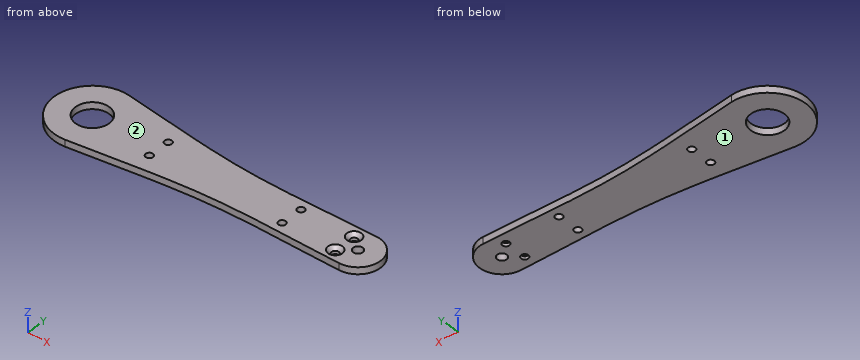
from build123d import *

# Parameters (mm, degrees)
SKETCH1_R           = 7.5
SKETCH1_R_2         = 2.125
SKETCH1_R_3         = 1.6
BOSS_EXTRUDE1_DEPTH = 3
SKETCH2_R           = 1.6
CUT_EXTRUDE1_DEPTH  = 79.91134278
CHAMFER1_SIZE       = 1.6


with BuildPart() as part:
    # Sketch1 → Boss-Extrude1 (new body)
    with BuildSketch(Plane.XY):
        with BuildLine():
            ThreePointArc((-57.956829007, 16.876772567), (-77, 0), (-57.956829007, -16.876772567))
            add(Edge.make_bspline(
                [(60, -10), (39.938279517, -10), (0.415985338, -7.693613776), (-38.598478023, -14.486949791), (-57.956829007, -16.876772567)],
                knots=[0, 0, 0, 0, 0.506913544, 1, 1, 1, 1], degree=3))
            ThreePointArc((60, -10), (70, 0), (60, 10))
            add(Edge.make_bspline(
                [(60, 10), (39.938279517, 10), (0.415985338, 7.693613776), (-38.598478023, 14.486949791), (-57.956829007, 16.876772567)],
                knots=[0, 0, 0, 0, 0.506913544, 1, 1, 1, 1], degree=3))
        make_face()
        with Locations((-60, 0)):
            Circle(SKETCH1_R, mode=Mode.SUBTRACT)
        with Locations(Location((60, 0, 0), (0, 0, 180))):
            Circle(SKETCH1_R_2, mode=Mode.SUBTRACT)
        with Locations((-30, 5)):
            Circle(SKETCH1_R_3, mode=Mode.SUBTRACT)
        with Locations((30, 5)):
            Circle(SKETCH1_R_3, mode=Mode.SUBTRACT)
        with Locations((30, -5)):
            Circle(SKETCH1_R_3, mode=Mode.SUBTRACT)
        with Locations((-30, -5)):
            Circle(SKETCH1_R_3, mode=Mode.SUBTRACT)
    extrude(amount=BOSS_EXTRUDE1_DEPTH)

    # Sketch2 → Cut-Extrude1 (cut, through all)
    with BuildSketch(Plane.XY.offset(3)):
        with Locations((54, 5)):
            Circle(SKETCH2_R)
        with Locations(Location((54, -5, 0), (0, 0, 180))):
            Circle(SKETCH2_R)
    extrude(amount=-CUT_EXTRUDE1_DEPTH, mode=Mode.SUBTRACT)

    # Chamfer1
    chamfer1_edges = [part.edges().sort_by_distance(p)[0] for p in [
        (52.4, 5, 3),
        (55.6, -5, 3),
    ]]
    chamfer(chamfer1_edges, length=CHAMFER1_SIZE)


solid = part.part
The model under review builds one solid part; all positions refer to its coordinate system, in mm. Face numbers are marked on the shaded views. Give positions to 0.01 mm unless a question says otherwise; leave off trailing zeros. Loops run counter-clockwise (first coordinate to the right, second up) from the corner with the lowest first, then second, coordinate; pieces in that order, holes last. Notation, with made-up numbers: (16.25, -9) -> (32.25, -9) arc R11 cw to (32.25, -4) -> close; hole circle Ø1 at (45.25, 26). An arc over 180 degrees is marked (long way). Put each result on its own line as item: value. Start each with the question number.
1. Mouldability with a two-part tool opening along Z and no side actions: class the marked faces 1 and 2 as released by +Z, released by -Z, zero draft, split by the parting line, or undercut.
2. We need section A-A on y = 0. State the section outline as (x, z) points (3 decimals), then the cut area to 3 significant figures.
3. Clearance check with flat-ended pins moving along their axes: P1, Ø3, axis at x = -30, y = 5, coming from the +Z side; P2, Ø3.5, axis at x = 54, y = 5, coming from the +Z side; P3, Ø1, axis at y = -8.5, z = 2.5, coming from the -X side; P4, Ø5, axis at x = 54, y = -5, coming from the +Z side. State where each tip first meets the part, or that it passes through.
4. We need section B-B on x = -60. State the section outline as (y, z) points.
5. Wall thickness on probe 1 along Y at (x, z) = (-30, 2.3); probe 2 along Y at (x, z) = (30, 0.75); probe 3 along X at (y, z) = (0.5, 1.6): over which ranges is each line inside the solid? List them lowest first.
6. We need section C-C on z = 0.7. State how many separate pieces and enclosed holes the cut face has, then the cut area to 3 significant figures.
Determined:
1. face 1: released by -Z
1. face 2: released by +Z
2. outline: (-77, 0) -> (-67.5, 0) -> (-67.5, 3) -> (-77, 3) -> close; (-52.5, 0) -> (57.875, 0) -> (57.875, 3) -> (-52.5, 3) -> close; (62.125, 0) -> (70, 0) -> (70, 3) -> (62.125, 3) -> close
2. area: 383 mm^2
3. P1: through
3. P2: z = 1.55
3. P3: x = -75
3. P4: z = 2.3
4. outline: (-17, 0) -> (-7.5, 0) -> (-7.5, 3) -> (-17, 3) -> close; (7.5, 0) -> (17, 0) -> (17, 3) -> (7.5, 3) -> close
5. probe 1: -13.1 to -6.6, -3.4 to 3.4, 6.6 to 13.1
5. probe 2: -9.56 to -6.6, -3.4 to 3.4, 6.6 to 9.56
5. probe 3: -76.99 to -67.48, -52.52 to 57.93, 62.07 to 69.99
6. separate pieces: 1
6. enclosed holes: 8
6. area: 3,130 mm^2
